Read the model definition and answer for the solid it produces. Units are mm, in the model's axes. Give positions to 0.01 mm unless a question says otherwise; leave off trailing zeros. Write each loop counter-clockwise with the first axis right and the second up, starting at its lowest first coordinate (ties: lowest second). Pieces come first, ordered by that corner, then holes. Notation, with made-up numbers: (-1.5, 35.25) - (13.5, 35.25) arc R14 ccw to (13.5, 59.25) - close; hole circle Ø4 at (5.25, 70). An arc over 180 degrees is marked (long way). Use CSV: the item, a comma, the result in double quotes. Start each with the question number.
from build123d import *

# Parameters (mm, degrees)
F0_W     = 10
F0_H     = 20
F1_DEPTH = 101.6
F2_R     = 6.35
F2_R_2   = 20
F3_DEPTH = 25.4
F4_R     = 9.99999


# Not quite as in the source:
# - a fillet or chamfer is up to 0.001 mm smaller than in the source, because OpenCascade refuses the exact size


with BuildPart() as f1:
    # F0 (on Top) → F1 (new body)
    with BuildSketch(Plane.XY):
        with Locations((5, -10)):
            Rectangle(F0_W, F0_H)
    extrude(amount=F1_DEPTH)

    # F2 (on face) → F3 (cut)
    with BuildSketch(Plane(origin=(0, 0, 0), x_dir=(0, -1, 0), z_dir=(-1, 0, 0))):
        with Locations((10, 10)):
            Circle(F2_R)
        with Locations((10, 118.9205080757)):
            Circle(F2_R_2)
    extrude(amount=-F3_DEPTH, mode=Mode.SUBTRACT)

    # F4 (radius 10 in the source; OpenCascade refuses exactly that, so slightly less here)
    f4_edges = [f1.edges().sort_by_distance(p)[0] for p in [
        (5, -20, 0),
        (5, 0, 0),
    ]]
    fillet(f4_edges, radius=F4_R)


solid = f1.part
(1) Given P1, Ø3, axis at x = 1.5, y = -13, coming from the +Z side; P2, Ø2, axis at x = 4, y = -7, coming from the +Z side; P3, Ø3, axis at x = 2, y = -9.5, coming from the +Z side, each flat-ended and moving along its own axis, determine where each tip first touches the part or whether it passes through.
(2) The part is cut by section B-B on y = -15.25. Write down the section's boundary in (x, z).
(3) Consider probe 1 along Z at (x, y) = (5.25, -10); probe 2 along Z at (x, y) = (7.5, -8.5); probe 3 along Z at (x, y) = (7.5, -19). Determine where each line is inside the solid, lowest interval first.
(4) For a pull along Y with two mould halves and no side action, classify faces 1 (the face through (4.93, -9.85, 98.92)), 2 (the face through (10, -10, 50)), 3 (the face through (5.07, -16.99, 2.85)) as pulls with the +Y half, pulls with the -Y half, needs draft (parallel to the pull), parting line crosses it, or undercut.
(5) The part is cut by section C-C on y = -6.25. Write down the section's boundary in (x, z), plus the area to 3 significant figures.
Reported:
1,P1,"z = 99.43"
1,P2,"z = 99.32"
1,P3,"z = 99.02"
2,outline,"(0, 1.49) - (10, 1.49) - (10, 6.43) - (0, 6.43) - close; (0, 13.57) - (10, 13.57) - (10, 99.62) - (0, 99.62) - close"
3,probe 1,"0 to 3.65, 16.35 to 98.92"
3,probe 2,"0.11 to 3.83, 16.17 to 98.98"
3,probe 3,"5.64 to 101.06"
4,face 1,"undercut"
4,face 2,"needs draft"
4,face 3,"pulls with the -Y half"
5,outline,"(0, 0.73) - (10, 0.73) - (10, 4.88) - (0, 4.88) - close; (0, 15.12) - (10, 15.12) - (10, 99.28) - (0, 99.28) - close"
5,area,"883 mm²"
